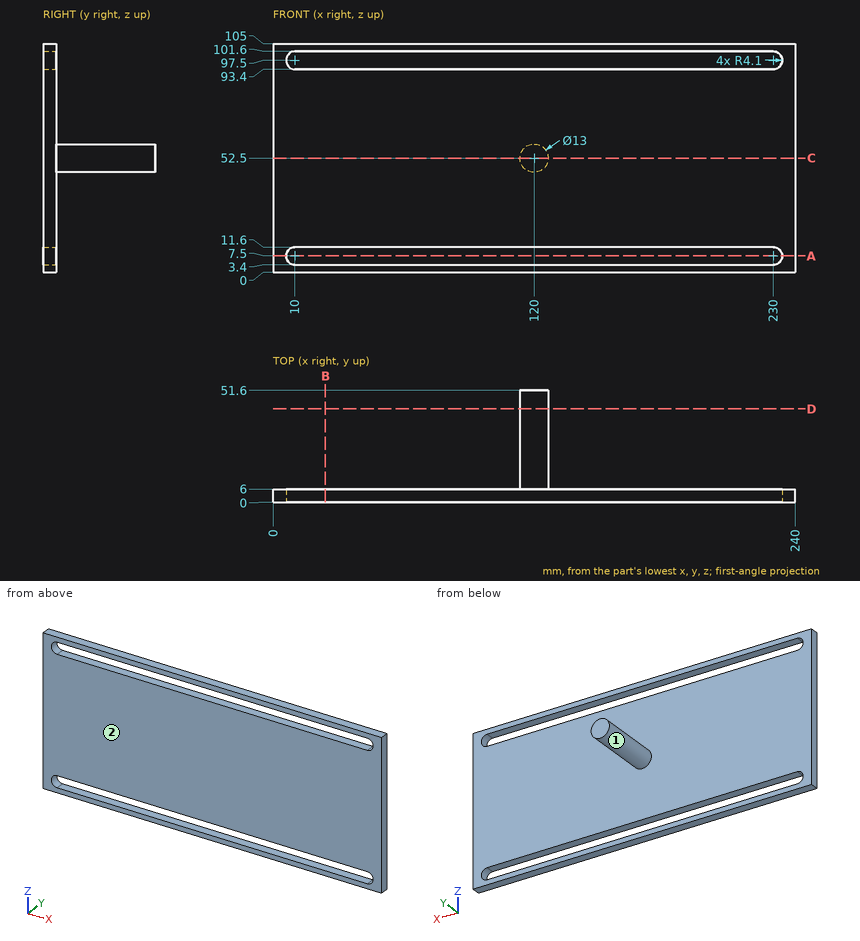
Job drawing, mm, ordinate dimensions from the low corner. One solid piece. A direction names the side the tool comes from. Give positions to 0.01 mm unless a question says otherwise; leave off trailing zeros. Loops run counter-clockwise (first coordinate to the right, second up) from the corner with the lowest first, then second, coordinate; pieces in that order, holes last. Notation, with made-up numbers: (80, -33) -> (101, -33) arc R20 ccw to (101, -15) -> close; hole circle Ø6 at (29.5, 40). An arc over 180 degrees is marked (long way). Write each question's results on one line, items separated by ' | '.
(1) Flat gauge pins, fed straight in: pin 1 Ø5 at (x, y) = (100, 9) entering from -Z; pin 2 Ø6 at (y, z) = (32, 52) entering from +X. Where does each tip first touch, or does it go through?
Geometry results:
pin 1: passes through | pin 2: stops at x = 126.5
(2) Cut at A-A on z = 7.5. List the corners of the cut face in (x, y), and give its area (3 significant figures).
Geometry results:
outline: (0, 0) -> (5.9, 0) -> (5.9, 6) -> (0, 6) -> close; (234.1, 0) -> (240, 0) -> (240, 6) -> (234.1, 6) -> close | area: 70.8 mm²
(3) Cut at C-C on z = 52.5. List the corners of the cut face in (x, y), and give its area (3 significant figures).
Geometry results:
outline: (0, 0) -> (240, 0) -> (240, 6) -> (126.5, 6) -> (126.5, 51.6) -> (113.5, 51.6) -> (113.5, 6) -> (0, 6) -> close | area: 2,030 mm²
(4) Cut at B-B on x = 24. List the corners of the cut face in (y, z), and give its area (3 significant figures).
Geometry results:
outline: (0, 0) -> (6, 0) -> (6, 3.4) -> (0, 3.4) -> close; (0, 11.6) -> (6, 11.6) -> (6, 93.4) -> (0, 93.4) -> close; (0, 101.6) -> (6, 101.6) -> (6, 105) -> (0, 105) -> close | area: 532 mm²
(5) Tool access for the marked faces 1 and 2: list every direction of +Z, -Z, +X, -X, +Y, -Y with a clear straight run to the whole face (end or side of a thin tool).
Geometry results:
face 1: +Y | face 2: +Z, -Z, +X, -X, -Y
(6) Cut at D-D on y = 43. List the corners of the cut face in (x, z), and give its area (3 significant figures).
Geometry results:
outline: circle Ø13 at (120, 52.5) | area: 133 mm²
(7) Probe line 1 along Z through (x, y) = (155.5, 5); line 2 along Y through (x, z) = (151, 35); line 3 along X through (y, z) = (45, 52). List the from-to ranges inside material, lowest first.
Geometry results:
line 1: z = 0 to 3.4, 11.6 to 93.4, 101.6 to 105 | line 2: y = 0 to 6 | line 3: x = 113.52 to 126.48
